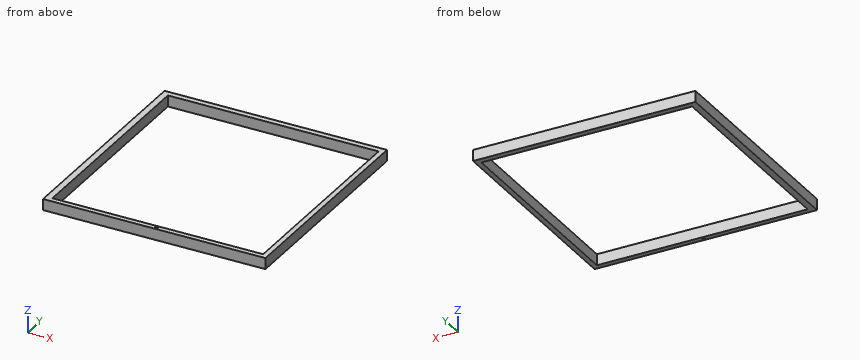
```python
from build123d import *

# Parameters (mm, degrees)
F0_W     = 25.4
F0_H     = 254
F1_DEPTH = 5.08
F5_W     = 508
F5_H     = 508
F5_W_2   = 481.2670946121
F5_H_2   = 482.8459620476
F6_DEPTH = 25.4
F9_D     = 6.35


with BuildPart() as f1:
    # F0 (on Top) → F1 (new body)
    with BuildSketch(Plane.XY):
        with Locations((-293.8296190764, 14.3110007048)):
            Rectangle(F0_W, F0_H)
    extrude(amount=F1_DEPTH)


with BuildPart() as f6:
    # F5 (on face) → F6 (new body)
    with BuildSketch(Plane.XY):
        with Locations((-1557.362942471, 41.7894273996)):
            Rectangle(F5_W, F5_H)
        with Locations((-1555.7374358177, 40.9697592258)):
            Rectangle(F5_W_2, F5_H_2, mode=Mode.SUBTRACT)
    extrude(amount=F6_DEPTH)

    # F9 (through all)
    with Locations(Plane(origin=(0, 0, 0), x_dir=(1, 0, 0), z_dir=(0, 0, -1))):
        with Locations((-1555.3545951843, 207.7113389969)):
            Hole(F9_D / 2)


solid = f6.part
```
Geometry: final body of the model. Coordinates: model frame, mm. Coordinates: 2 decimals unless noted, no trailing zeros. Order: outer loops, then holes, each group sorted by start corner. A loop starts at its lowest first (then second) coordinate and runs counter-clockwise, first axis right, second up. Notation, with made-up numbers: (74.25, 76) -> (92.25, 76) arc R8 cw to (92.25, 82) -> close; hole circle Ø2 at (49.25, 12). An arc over 180 degrees is marked (long way). Write item = value, one per line.
(1) Pin query (flat end, axial travel): pin 1 Ø5 at (x, y) = (-1555.35, -207.71) entering from +Z. Return the tip coordinate at first contact, or that it passes through.
Solved:
pin_1 = through
(2) Line query: line 1 (X direction, y = -143.5, z = 20); line 2 (Y direction, x = -1650, z = 22.5). Output: solid intervals per line, ascending.
Solved:
line_1 = -1811.36 to -1796.37, -1315.1 to -1303.36
line_2 = -212.21 to -200.45, 282.39 to 295.79
(3) Cut plane C-C on z = 13.75. Return loops of the section in (x, y) (3 decimals), plus the area to 3 significant figures.
Solved:
outline = (-1811.363, -212.211) -> (-1303.363, -212.211) -> (-1303.363, 295.789) -> (-1811.363, 295.789) -> close; hole (-1796.371, -200.453) -> (-1315.104, -200.453) -> (-1315.104, 282.393) -> (-1796.371, 282.393) -> close; hole circle Ø6.35 at (-1555.355, -207.711)
area = 25,700 mm²
(4) Cut plane B-B on y = -146.5. Return loops of the section in (x, z).
Solved:
outline = (-1811.36, 0) -> (-1796.37, 0) -> (-1796.37, 25.4) -> (-1811.36, 25.4) -> close; (-1315.1, 0) -> (-1303.36, 0) -> (-1303.36, 25.4) -> (-1315.1, 25.4) -> close
(5) Cut plane A-A on x = -1414. Return loops of the section in (y, z).
Solved:
outline = (-212.21, 0) -> (-200.45, 0) -> (-200.45, 25.4) -> (-212.21, 25.4) -> close; (282.39, 0) -> (295.79, 0) -> (295.79, 25.4) -> (282.39, 25.4) -> close
